Here's how the part is built. I have some questions about the finished solid (model axes, mm). Face numbers are marked on the shaded views. A direction names the side the tool comes from. Give positions to 0.01 mm unless a question says otherwise; leave off trailing zeros. Loops run counter-clockwise (first coordinate to the right, second up) from the corner with the lowest first, then second, coordinate; pieces in that order, holes last.
Q1. Suppose I cut it at B-B (y = 0). List the corners of the cut face in (x, z) for me.
Q2. Suppose I cut it at D-D (y = -2.05). List the corners of the cut face in (x, z) for me, and give its area (3 significant figures).
Q3. I'm going to push flat-ended pins straight in: P1, Ø1.6, axis at x = -3.5, y = -0.5, coming from the -Z side; P2, Ø1.5, axis at y = 2, z = -1, coming from the -X side; P3, Ø0.8, axis at x = 0, y = -1.5, coming from the +Z side. Where does each tip first touch, or does it pass through?
Q4. Suppose I cut it at C-C (x = -1.75). List the corners of the cut face in (y, z) for me, and give its area (3 significant figures).
Q5. I need wall thicknesses on probe 1 along Y at (x, z) = (0, -1.6); probe 2 along Z at (x, y) = (-4.5, 0.2); probe 3 along Z at (x, y) = (-1.25, -1.4). Which ranges of each line are inside material? Lowest first, please.
Q6. Suppose I cut it at A-A (x = 3.5). List the corners of the cut face in (y, z) for me.
Q7. For the marked faces 1, 2 and 3, which set-ups out of +Z, -Z, +X, -X, +Y, -Y let a thin tool reach every point of the face, with its end or its side?
Q8. Thinking about a two-plate mould opening in Y: for the marked faces 4, 5, 6 and 7, which applies, pulls with the +Y half, pulls with the -Y half, needs draft (parallel to the pull), parting line crosses it, or undercut?
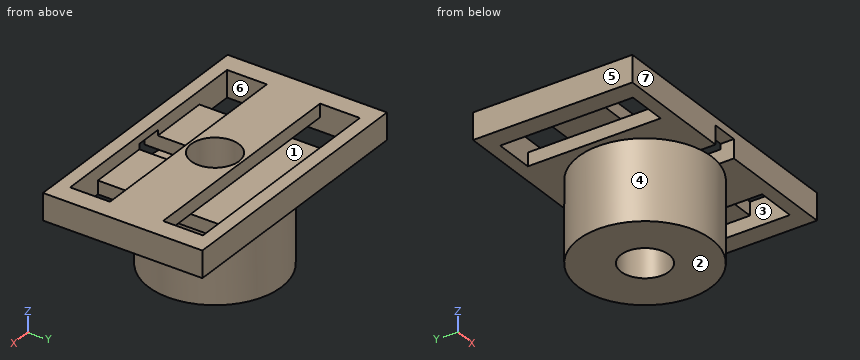
```python
from build123d import *

# Parameters (mm, degrees)
F0_W      = 10
F0_H      = 6
F0_W_2    = 1.5
F0_H_2    = 5
F1_DEPTH  = 0.5
F2_W      = 10
F2_H      = 6
F3_DEPTH  = 0.5
F5_DEPTH  = 0.5
F6_W      = 1
F6_H      = 0.5
F7_DEPTH  = 2
F8_R      = 2.5
F8_R_2    = 0.9
F9_DEPTH  = 3
F10_R     = 0.9
F11_DEPTH = 4.001
F12_DEPTH = 0.2


with BuildPart() as f1:
    # F0 (on Top) → F1 (new body)
    with BuildSketch(Plane.XY):
        Rectangle(F0_W, F0_H)
        with Locations((-3.5, 0)):
            Rectangle(F0_W_2, F0_H_2, mode=Mode.SUBTRACT)
        with Locations((3.5, 0)):
            Rectangle(F0_W_2, F0_H_2, mode=Mode.SUBTRACT)
    extrude(amount=F1_DEPTH)

    # F2 (on face) → F3 (join)
    with BuildSketch(Plane.XY.offset(0.5)):
        Rectangle(F2_W, F2_H)
    extrude(amount=F3_DEPTH)

    # F4 (on face) → F5 (cut)
    with BuildSketch(Plane.XY.offset(1)):
        Polygon((-4.25, -1), (-4.25, -2.5), (-2.75, -2.5), (2.75, -2.5), (4.25, -2.5), (4.25, -1), align=None)
        Polygon((-4.25, 2.5), (-4.25, 1), (4.25, 1), (4.25, 2.5), (2.75, 2.5), (-2.75, 2.5), align=None)
    extrude(amount=-F5_DEPTH, mode=Mode.SUBTRACT)

    # F6 (on face) → F7 (cut, through all)
    with BuildSketch(Plane.XZ.offset(3)):
        with Locations((0, 0.45)):
            Rectangle(F6_W, F6_H)
    extrude(amount=-F7_DEPTH, mode=Mode.SUBTRACT)

    # F8 (on face) → F9 (join)
    with BuildSketch(Plane.XY):
        Circle(F8_R)
        Circle(F8_R_2, mode=Mode.SUBTRACT)
    extrude(amount=-F9_DEPTH)

    # F10 (on face) → F11 (cut, through all)
    with BuildSketch(Plane.XY.offset(1)):
        Circle(F10_R)
    extrude(amount=-F11_DEPTH, mode=Mode.SUBTRACT)

    # F12 (cut, through all): a face of the model
    f12_faces = [f1.faces().sort_by_distance(p)[0] for p in [
        (0, -2, 0.2),
    ]]
    extrude(f12_faces, amount=-F12_DEPTH, mode=Mode.SUBTRACT)


solid = f1.part
```
Solutions:
1. outline: (-5, 0) - (-4.25, 0) - (-4.25, 0.5) - (-2.75, 0.5) - (-2.75, 0) - (-2.5, 0) - (-2.5, -3) - (-0.9, -3) - (-0.9, 1) - (-5, 1) - close; (0.9, -3) - (2.5, -3) - (2.5, 0) - (2.75, 0) - (2.75, 0.5) - (4.25, 0.5) - (4.25, 0) - (5, 0) - (5, 1) - (0.9, 1) - close
2. outline: (-5, 0) - (-4.25, 0) - (-4.25, 1) - (-5, 1) - close; (-2.75, 0) - (-1.43, 0) - (-1.43, -3) - (1.43, -3) - (1.43, 0) - (2.75, 0) - (2.75, 0.5) - (0.5, 0.5) - (0.5, 0) - (-0.5, 0) - (-0.5, 0.5) - (-2.75, 0.5) - close; (4.25, 0) - (5, 0) - (5, 1) - (4.25, 1) - close
2. area: 12.3 mm2
3. P1: stops at z = 0
3. P2: stops at x = -2.17
3. P3: stops at z = 0
4. outline: (-3, 0) - (-1.79, 0) - (-1.79, -3) - (1.79, -3) - (1.79, 0) - (3, 0) - (3, 1) - (2.5, 1) - (2.5, 0.5) - (1, 0.5) - (1, 1) - (-1, 1) - (-1, 0.5) - (-2.5, 0.5) - (-2.5, 1) - (-3, 1) - close
4. area: 15.2 mm2
5. probe 1: y = -2.5 to -0.9, 0.9 to 2.5
5. probe 2: z = 0 to 1
5. probe 3: z = -3 to 0.5
6. outline: (-3, 0) - (-2.5, 0) - (-2.5, 1) - (-3, 1) - close; (-1, 0.5) - (1, 0.5) - (1, 1) - (-1, 1) - close; (2.5, 0) - (3, 0) - (3, 1) - (2.5, 1) - close
7. face 1: +Z
7. face 2: -Z, +X, -X, +Y, -Y
7. face 3: -Z
8. face 4: parting line crosses it
8. face 5: needs draft
8. face 6: undercut
8. face 7: pulls with the -Y half
